The listing builds one solid part. Answer for the finished solid, in the listing's coordinates (mm). Coordinates: 2 decimals unless noted, no trailing zeros. Loops run counter-clockwise (first coordinate to the right, second up) from the corner with the lowest first, then second, coordinate; pieces in that order, holes last. Notation, with made-up numbers: (29.5, 5.5) -> (86.5, 5.5) arc R10 ccw to (86.5, 11.5) -> close; hole circle Ø11 at (-4, 30). An arc over 180 degrees is marked (long way). Answer in a Markdown table with one row per item.
```python
from build123d import *

# Parameters (mm, degrees)
SKETCH1_R          = 1.5
SKETCH1_RX         = 1.5
SKETCH1_RY         = 1.499999958
BASE_FLANGE1_DEPTH = 3.175
SKETCH2_R          = 3.15
CUT_EXTRUDE1_DEPTH = 10


# Sheet-metal steps are written as plain solids
with BuildPart() as part:
    # Sketch1 → Base-Flange1 (new body)
    with BuildSketch(Plane(origin=(0, 0, 0), x_dir=(0, 0, -1), z_dir=(1, 0, 0))):
        with BuildLine():
            Line((15.865201272, 80.394978876), (48.626542571, 80.394978876))
            ThreePointArc((48.626542571, 80.394978876), (52.162076477, 78.930512782), (53.626542571, 75.394978876))
            Line((53.626542571, 75.394978876), (53.626542571, 43.023123453))
            ThreePointArc((53.626542571, 43.023123453), (53.381665801, 41.477548132), (52.671021343, 40.083363009))
            Line((52.671021343, 40.083363009), (24.97388681, 1.978056535))
            ThreePointArc((24.97388681, 1.978056535), (23.188445465, 0.457239672), (20.905954013, -0.082128012))
            Line((20.905954013, -0.082128012), (6.9504e-05, 0.015938493))
            Line((6.9504e-05, 0.015938493), (0.167574588, 38.427897973))
            Line((0.167574588, 38.427897973), (-38.331753926, 38.667513874))
            Line((-38.331753926, 38.667513874), (-38.283953708, 49.628972315))
            ThreePointArc((-38.283953708, 49.628972315), (-37.557098456, 52.203443057), (-35.60707457, 54.034733587))
            Line((-35.60707457, 54.034733587), (13.54212795, 79.822543708))
            ThreePointArc((13.54212795, 79.822543708), (14.668920402, 80.249761269), (15.865201272, 80.394978876))
        make_face()
        with Locations((17.130255889, 43.891226665)):
            Circle(SKETCH1_R, mode=Mode.SUBTRACT)
        with Locations(Location((48.129224581, 43.894326732), (0, 0, 119.309738267))):
            Ellipse(SKETCH1_RX, SKETCH1_RY, mode=Mode.SUBTRACT)
        with Locations(Location((17.126576602, 74.891226239), (0, 0, 119.309738267))):
            Ellipse(SKETCH1_RX, SKETCH1_RY, mode=Mode.SUBTRACT)
        with Locations(Location((48.126575725, 74.894904787), (0, 0, 119.309738267))):
            Ellipse(SKETCH1_RX, SKETCH1_RY, mode=Mode.SUBTRACT)
        with BuildLine():
            add(Edge.make_bspline(
                [(32.302616578, 47.592077565), (33.84702501, 47.592261157), (36.935768822, 48.207032249), (40.863315512, 50.83201062), (43.487359793, 54.760181559), (44.408414716, 59.393516648), (43.486258021, 64.026632625), (40.861279703, 67.954179586), (36.93310891, 70.578224108), (32.299774036, 71.499279195), (27.666658318, 70.577122557), (23.739111629, 67.952144186), (21.115067347, 64.023973247), (20.194012424, 59.390638157), (21.116169119, 54.75752218), (23.741147438, 50.82997522), (27.669318231, 48.205930698), (30.758208146, 47.591893973), (32.302616578, 47.592077565)],
                knots=[0, 0, 0, 0, 0.392699082, 0.785398163, 1.178097245, 1.570796327, 1.963495408, 2.35619449, 2.748893572, 3.141592654, 3.534291735, 3.926990817, 4.319689899, 4.71238898, 5.105088062, 5.497787144, 5.890486225, 6.283185307, 6.283185307, 6.283185307, 6.283185307], degree=3))
        make_face(mode=Mode.SUBTRACT)
    extrude(amount=-BASE_FLANGE1_DEPTH)

    # Sketch2 → Cut-Extrude1 (cut)
    with BuildSketch(Plane(origin=(-3.175, -854.244613751, -1311.587435239), x_dir=(0, 0, 1), z_dir=(-1, 0, 0))):
        with Locations((1283.833112159, 884.130691082)):
            Circle(SKETCH2_R)
        with Locations((1298.892990926, 864.201114773)):
            Circle(SKETCH2_R)
        with Locations((1341.343837435, 904.15787978)):
            Circle(SKETCH2_R)
        with Locations((1321.311357388, 911.570594384)):
            Circle(SKETCH2_R)
    extrude(amount=-CUT_EXTRUDE1_DEPTH, mode=Mode.SUBTRACT)


solid = part.part
```
Item 1: Flat-ended cylindrical pins translate along their axes: pin 1 Ø5.5 at (y, z) = (29.89, -27.75) entering from -X; pin 2 Ø1 at (x, y) = (-2, 60.5) entering from +Z. Find the tip coordinate at first contact, or state that the pin passes through.
Findings below:
| item | result |
|---|---|
| pin 1 | passes through |
| pin 2 | stops at z = 24.24 |
Item 2: A cutting plane is placed at C-C, the plane x = -2.15. Count the separate pieces of the cut face and the enclosed holes in it, plus the area to 3 significant figures.
Findings below:
| item | result |
|---|---|
| separate pieces | 1 |
| enclosed holes | 9 |
| area | 3,960 mm2 |
Item 3: A cutting plane is placed at D-D, the plane z = -3. Determine the outline of the cut face in (x, y) (3 decimals).
Findings below:
| item | result |
|---|---|
| outline | (-3.175, 0.002) -> (0, 0.002) -> (0, 74.291) -> (-3.175, 74.291) -> close |
Item 4: A cutting plane is placed at A-A, the plane z = 28. Determine the outline of the cut face in (x, y) (3 decimals).
Findings below:
| item | result |
|---|---|
| outline | (-3.175, 38.603) -> (0, 38.603) -> (0, 47.298) -> (-3.175, 47.298) -> close; (-3.175, 52.528) -> (0, 52.528) -> (0, 58.026) -> (-3.175, 58.026) -> close |
Item 5: A cutting plane is placed at B-B, the plane y = 25. Determine the outline of the cut face in (x, z) (3 decimals).
Findings below:
| item | result |
|---|---|
| outline | (-3.175, -41.708) -> (0, -41.708) -> (0, -0.109) -> (-3.175, -0.109) -> close |
Item 6: Find the intervals of material crossed by probe 1 along Z at (x, y) = (-1.5, 44); probe 2 along Y at (x, z) = (-2.7, -27); probe 3 along Z at (x, y) = (-2.25, 74.5), in increasing order.
Findings below:
| item | result |
|---|---|
| probe 1 | z = -53.63 to -49.63, -46.63 to -18.63, -15.63 to 38.31 |
| probe 2 | y = 4.77 to 26.83, 32.94 to 48.85, 69.93 to 80.39 |
| probe 3 | z = -53.63 to -49.57, -46.68 to -18.57, -15.68 to -3.4 |
Item 7: Determine the mould class of faces 1 (the face through (-1.61, 26.81, -28.44)), 2 (the face through (-1.57, 41.5, -53.39)), 3 (the face through (-1.565, 80.246, -14.653)) for opening direction Z: +Z half, -Z half, draft (parallel to the pull), parting line (faces both ways), or undercut.
Findings below:
| item | result |
|---|---|
| face 1 | undercut |
| face 2 | -Z half |
| face 3 | +Z half |
